```python
from build123d import *

# Parameters (mm, degrees)
F4_DEPTH  = 2.205
F4_TAPER  = 10
F5_W      = 2.995
F5_H      = 0.9355060756
F5_H_2    = 2.985
F5_W_2    = 2.4
F6_DEPTH  = 0.585
F7_W      = 19.795
F7_H      = 26.085
F8_DEPTH  = 2.795
F8_TAPER  = 10
F9_W      = 1.17
F9_H      = 0.585
F10_DEPTH = 6


with BuildPart() as f4:
    # F3 (on Top) → F4 (new body)
    with BuildSketch(Plane.XY):
        with BuildLine():
            Line((9.8975, 21.9575), (9.8975, 26.085))
            Line((9.8975, 26.085), (-9.8975, 26.085))
            Line((-9.8975, 26.085), (-9.8975, 21.9575))
            ThreePointArc((-9.8975, 21.9575), (-7.725, 19.785), (-9.8975, 17.6125))
            Line((-9.8975, 17.6125), (-9.8975, 12.33))
            ThreePointArc((-9.8975, 12.33), (-8.7675, 11.2), (-9.8975, 10.07))
            Line((-9.8975, 10.07), (-9.8975, 0))
            Line((-9.8975, 0), (9.8975, 0))
            Line((9.8975, 0), (9.8975, 10.07))
            ThreePointArc((9.8975, 10.07), (8.7675, 11.2), (9.8975, 12.33))
            Line((9.8975, 12.33), (9.8975, 17.6125))
            ThreePointArc((9.8975, 17.6125), (7.725, 19.785), (9.8975, 21.9575))
        make_face()
    extrude(amount=F4_DEPTH, taper=F4_TAPER)

    # F5 (on face) → F6 (join)
    with BuildSketch(Plane.XY):
        with Locations((0, 0.4677530378)):
            Rectangle(F5_W, F5_H)
        with Locations((0, -1.4925)):
            Rectangle(F5_W, F5_H_2)
        with Locations((-5.46, 0.4677530378)):
            Rectangle(F5_W_2, F5_H)
        Polygon((-4.26, 0), (-6.66, 0), (-6.66, -2.4), (-6.045, -2.4), (-6.045, -2.985), (-4.875, -2.985), (-4.875, -2.4), (-4.26, -2.4), align=None)
        Polygon((4.875, -2.985), (6.045, -2.985), (6.045, -2.4), (6.66, -2.4), (6.66, 0), (4.26, 0), (4.26, -2.4), (4.875, -2.4), align=None)
        with Locations((5.46, 0.4677530378)):
            Rectangle(F5_W_2, F5_H)
    extrude(amount=F6_DEPTH)

    # F7 (on face) → F8 (join)
    with BuildSketch(Plane.XY):
        with Locations((0, 13.0425)):
            Rectangle(F7_W, F7_H)
    extrude(amount=-F8_DEPTH, taper=F8_TAPER)

    # F9 (on face) → F10 (join)
    with BuildSketch(Plane(origin=(0, 0, 0), x_dir=(1, 0, 0), z_dir=(0, 0, -1))):
        with Locations((0, 2.6925)):
            Rectangle(F9_W, F9_H)
        with Locations((-5.46, 2.6925)):
            Rectangle(F9_W, F9_H)
        with Locations((5.46, 2.6925)):
            Rectangle(F9_W, F9_H)
    extrude(amount=F10_DEPTH)


solid = f4.part
```
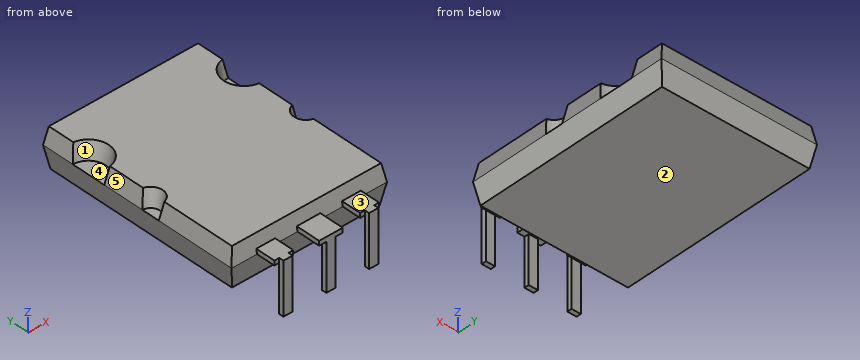
The listing builds one solid part. Answer for the finished solid, in the listing's coordinates (mm). Face numbers are marked on the shaded views. A direction names the side the tool comes from. Round coordinates to 2 decimals unless told otherwise and drop trailing zeros. Order: outer loops, then holes, each group sorted by start corner. A loop starts at its lowest first (then second) coordinate and runs counter-clockwise, first axis right, second up. Notation, with made-up numbers: (60.5, 38) -> (103.5, 38) arc R9 ccw to (103.5, 51) -> close; hole circle Ø5 at (37.25, -24). An arc over 180 degrees is marked (long way). Answer as CSV lines item,"result". Start each with the question number.
(1) Flat-ended cylindrical pins translate along their axes: pin 1 Ø2 at (x, y) = (3, 10) entering from -Z (3 decimals); pin 2 Ø0.6 at (y, z) = (-1.5, 0) entering from +X; pin 3 Ø0.6 at (x, z) = (-6.5, 0) entering from -Y. Find the tip coordinate at first contact, or state that the pin passes through.
(2) For a pull along Y with two mould halves and no side action, classify the marked faces 1 and 2 as +Y half, -Y half, draft (parallel to the pull), parting line (faces both ways), or undercut.
(3) The part is cut by section B-B (z = -0.5). Count the separate pieces of the cut face and the enclosed holes in it, then the cut area to 3 significant figures.
(4) A tool of negligible diameter and unlimited length cuts with its end or side. For the marked faces 3, 4 and 5, from which of +Z, -Z, +X, -X, +Y, -Y can it reach the whole face along a straight path? Write none if from no direction.
(5) The part is cut by section A-A (z = 1.25). Determine the outline of the cut face in (x, y) (1 decimal), then the cut area to 3 significant figures.
(6) Find the intervals of material crossed by probe 1 along Z at (x, y) = (-7.75, 3.5) (3 decimals); probe 2 along Y at (x, z) = (-7.75, -2.25); probe 3 along Y at (x, z) = (-1.25, -2.75), in increasing order. Write a range as from..to.
Evaluation:
1,pin 1,"z = -2.795"
1,pin 2,"x = 6.66"
1,pin 3,"y = -2.4"
2,face 1,"undercut"
2,face 2,"draft"
3,separate pieces,"4"
3,enclosed holes,"0"
3,area,"510 mm²"
4,face 3,"+Z, +X, -X, -Y"
4,face 4,"+Z, -X"
4,face 5,"+Z, -X, +Y, -Y"
5,outline,"(-9.7, 0.2) -> (9.7, 0.2) -> (9.7, 9.9) arc R1.4 cw to (9.7, 12.5) -> (9.7, 17.4) arc R2.4 cw to (9.7, 22.2) -> (9.7, 25.9) -> (-9.7, 25.9) -> (-9.7, 22.2) arc R2.4 cw to (-9.7, 17.4) -> (-9.7, 12.5) arc R1.4 cw to (-9.7, 9.9) -> close"
5,area,"476 mm²"
6,probe 1,"-2.795..2.205"
6,probe 2,"0.4..25.69"
6,probe 3,"0.48..25.6"
